from build123d import *

# Parameters (mm, degrees)
SKETCH2_W           = 23
SKETCH2_H           = 19
BOSS_EXTRUDE1_DEPTH = 3
SKETCH3_W           = 1
SKETCH3_H           = 19
SKETCH3_W_2         = 3
BOSS_EXTRUDE2_DEPTH = 5
BOSS_EXTRUDE3_DEPTH = 19
SKETCH5_R           = 1.75
CUT_EXTRUDE1_DEPTH  = 4
SKETCH6_R           = 3
CUT_EXTRUDE2_DEPTH  = 1.7
SKETCH7_W           = 17.6
SKETCH7_H           = 4.9
BOSS_EXTRUDE4_DEPTH = 1.4
SKETCH8_W           = 2.5
SKETCH8_H           = 0.9
BOSS_EXTRUDE5_DEPTH = 19
SKETCH9_W           = 1.4
SKETCH9_H           = 0.8
CUT_EXTRUDE3_DEPTH  = 20
BOSS_EXTRUDE6_DEPTH = 1.2
CUT_EXTRUDE4_REACH  = 28
SKETCH11_R          = 1.75
FILLET1_R           = 2
FILLET2_R           = 2


with BuildPart() as part:
    # Sketch2 → Boss-Extrude1 (new body)
    with BuildSketch(Plane(origin=(0, 0, 0), x_dir=(1, 0, 0), z_dir=(0, 1, 0))):
        with Locations((11.5, 9.5)):
            Rectangle(SKETCH2_W, SKETCH2_H)
    extrude(amount=BOSS_EXTRUDE1_DEPTH)

    # Sketch3 → Boss-Extrude2 (add)
    with BuildSketch(Plane(origin=(0, 3, 0), x_dir=(1, 0, 0), z_dir=(0, 1, 0))):
        with Locations((0.5, 9.5)):
            Rectangle(SKETCH3_W, SKETCH3_H)
        with Locations((3.9, 9.5)):
            Rectangle(SKETCH3_W_2, SKETCH3_H)
    extrude(amount=BOSS_EXTRUDE2_DEPTH)

    # Sketch4 → Boss-Extrude3 (add)
    with BuildSketch(Plane(origin=(0, 0, -19), x_dir=(-1, 0, 0), z_dir=(0, 0, -1))):
        Polygon((0, 0), (3, 0), (3, 8), (3, 11), (-0.95, 11), (-0.95, 10), (1.5, 10), (1.5, 8), (0, 8), align=None)
    extrude(amount=-BOSS_EXTRUDE3_DEPTH)

    # Sketch5 → Cut-Extrude1 (cut, through all)
    with BuildSketch(Plane(origin=(0, 3, 0), x_dir=(1, 0, 0), z_dir=(0, 1, 0))):
        with Locations((18.8, 9.5)):
            Circle(SKETCH5_R)
    extrude(amount=-CUT_EXTRUDE1_DEPTH, mode=Mode.SUBTRACT)

    # Sketch6 → Cut-Extrude2 (cut)
    with BuildSketch(Plane.XZ):
        with Locations((18.8, -9.5)):
            Circle(SKETCH6_R)
    extrude(amount=-CUT_EXTRUDE2_DEPTH, mode=Mode.SUBTRACT)

    # Sketch7 → Boss-Extrude4 (add)
    with BuildSketch(Plane(origin=(0, 3, 0), x_dir=(1, 0, 0), z_dir=(0, 1, 0))):
        with Locations((14.2, 2.45)):
            Rectangle(SKETCH7_W, SKETCH7_H)
        with Locations((14.2, 16.55)):
            Rectangle(SKETCH7_W, SKETCH7_H)
    extrude(amount=BOSS_EXTRUDE4_DEPTH)

    # Sketch8 → Boss-Extrude5 (add)
    with BuildSketch(Plane(origin=(0, 0, -19), x_dir=(-1, 0, 0), z_dir=(0, 0, -1))):
        with Locations((0.25, 8.45)):
            Rectangle(SKETCH8_W, SKETCH8_H)
    extrude(amount=-BOSS_EXTRUDE5_DEPTH)

    # Sketch9 → Cut-Extrude3 (cut, through all)
    with BuildSketch(Plane(origin=(0, 0, -19), x_dir=(-1, 0, 0), z_dir=(0, 0, -1))):
        with Locations((-1.7, 2.6)):
            Rectangle(SKETCH9_W, SKETCH9_H)
    extrude(amount=-CUT_EXTRUDE3_DEPTH, mode=Mode.SUBTRACT)

    # Sketch10 → Boss-Extrude6 (add)
    with BuildSketch(Plane.XY):
        Polygon((-1.5, 8.9), (-1.5, 10), (0.95, 10), (0.95, 11), (5.4, 8), (2.4, 8), (2.4, 2.2), (1, 2.2), (1, 8.9), align=None)
    extrude(amount=-BOSS_EXTRUDE6_DEPTH)

    # Sketch11 → Cut-Extrude4 (cut, up to next)
    with BuildSketch(Plane.ZY.offset(3), mode=Mode.PRIVATE) as cut_extrude4_sk1:
        with Locations((-9.5, 5)):
            Circle(SKETCH11_R)
    cut_extrude4_tool1 = extrude(cut_extrude4_sk1.sketch, amount=-CUT_EXTRUDE4_REACH, mode=Mode.PRIVATE) & part.part
    add(cut_extrude4_tool1.solids().sort_by_distance((-3, 5, -9.5))[0], mode=Mode.SUBTRACT)

    # Fillet1
    fillet1_edges = [part.edges().sort_by_distance(p)[0] for p in [
        (-3, 11, -9.5),
    ]]
    fillet(fillet1_edges, radius=FILLET1_R)

    # Fillet2
    fillet2_edges = [part.edges().sort_by_distance(p)[0] for p in [
        (-3, 0, -9.5),
    ]]
    fillet(fillet2_edges, radius=FILLET2_R)


solid = part.part
Read the model definition and answer for the solid it produces. Units are mm, in the model's axes. A direction names the side the tool comes from. Give positions to 0.01 mm unless a question says otherwise; leave off trailing zeros. Write each loop counter-clockwise with the first axis right and the second up, starting at its lowest first coordinate (ties: lowest second). Pieces come first, ordered by that corner, then holes. Notation, with made-up numbers: (50, 39) - (93, 39) arc R26 ccw to (93, 74) - close; hole circle Ø7 at (17.25, 75.5). An arc over 180 degrees is marked (long way). Use CSV: the item, a comma, the result in double quotes. Start each with the question number.
Item 1: Flat-ended cylindrical pins translate along their axes: P1, Ø1.8, axis at x = 20, z = -8.5, coming from the -Y side; P2, Ø3.5, axis at x = 4.5, z = -8.5, coming from the +Y side; P3, Ø6, axis at x = 3.5, y = 8.5, coming from the +Z side; P4, Ø7.5, axis at x = 14.5, z = -10, coming from the +Y side. Find the tip coordinate at first contact, or state that the pin passes through.
Item 2: The part is cut by section D-D, the plane x = 12.5. Give the vertices of the cut face in (y, z), and give its area (3 significant figures).
Item 3: For faces 1 (the flat face through (1, 7, -10)), 2 (the flat face through (14, 4.4, -2)), 3 (the flat face through (0.95, 10.5, -10.2)), 4 (the flat face through (14, 4, -14.1)), determine the directions among +Z, -Z, +X, -X, +Y, -Y from which every point of the face is accessible in a straight line to the end or side of a thin tool.
Item 4: The mould has two halves that part along X. Classify faces 5 (the flat face through (23, 2, -9)), 6 (the cylindrical face through (15.8, 0.8, -9.4)), 7 (the flat face through (0, 8.9, -10)): pulls with the +X half, pulls with the -X half, needs draft (parallel to the pull), parting line crosses it, or undercut.
Item 5: The part is cut by section C-C, the plane x = 18.8. Give the vertices of the cut face in (y, z).
Item 6: The part is cut by section A-A, the plane z = -9.5. Give the vertices of the cut face in (x, y).
Item 7: Consider line 1 (X direction, y = 2.45, z = -9.5); line 2 (Z direction, x = 18.8, y = 2.4); line 3 (Z direction, x = 18.8, y = 0.55). Determine where each line is inside the solid, lowest interval first.
Item 8: The part is cut by section B-B, the plane y = 5. Give the vertices of the cut face in (x, z), and give its area (3 significant figures).
Taken from the geometry:
1,P1,"y = 1.7"
1,P2,"y = 8"
1,P3,"z = 0"
1,P4,"y = 3"
2,outline,"(0, -19) - (4.4, -19) - (4.4, -14.1) - (3, -14.1) - (3, -4.9) - (4.4, -4.9) - (4.4, 0) - (0, 0) - close"
2,area,"70.7 mm2"
3,face 1,"-Z, +Y"
3,face 2,"+Z, -Z, +X, +Y"
3,face 3,"-Z, +X, +Y"
3,face 4,"+X, +Y"
4,face 5,"pulls with the +X half"
4,face 6,"undercut"
4,face 7,"needs draft"
5,outline,"(0, -19) - (4.4, -19) - (4.4, -14.1) - (3, -14.1) - (3, -11.25) - (1.7, -11.25) - (1.7, -12.5) - (0, -12.5) - close; (0, -6.5) - (1.7, -6.5) - (1.7, -7.75) - (3, -7.75) - (3, -4.9) - (4.4, -4.9) - (4.4, 0) - (0, 0) - close"
6,outline,"(-3, 2) arc R2 ccw to (-1, 0) - (15.8, 0) - (15.8, 1.7) - (17.05, 1.7) - (17.05, 3) - (5.4, 3) - (5.4, 8) - (2.4, 8) - (2.4, 2.2) - (1, 2.2) - (1, 3.25) - (-3, 3.25) - close; (-3, 6.75) - (1, 6.75) - (1, 8.9) - (-1.5, 8.9) - (-1.5, 10) - (0.95, 10) - (0.95, 11) - (-1, 11) arc R2 ccw to (-3, 9) - close; (20.55, 1.7) - (21.8, 1.7) - (21.8, 0) - (23, 0) - (23, 3) - (20.55, 3) - close"
7,line 1,"-3 to 1, 2.4 to 17.05, 20.55 to 23"
7,line 2,"-19 to -11.25, -7.75 to 0"
7,line 3,"-19 to -12.5, -6.5 to 0"
8,outline,"(-3, -19) - (1, -19) - (1, -11.25) - (-3, -11.25) - close; (-3, -7.75) - (1, -7.75) - (1, -1.2) - (2.4, -1.2) - (2.4, -19) - (5.4, -19) - (5.4, 0) - (-3, 0) - close"
8,area,"121 mm2"
